Part model, mm, in its own coordinate system. A direction names the side the tool comes from. Give positions to 0.01 mm unless a question says otherwise; leave off trailing zeros. Order: outer loops, then holes, each group sorted by start corner. A loop starts at its lowest first (then second) coordinate and runs counter-clockwise, first axis right, second up. Notation, with made-up numbers: (51, 32.5) - (75, 32.5) arc R12 ccw to (75, 42.5) - close; hole circle Ø10 at (75.5, 32). An arc over 180 degrees is marked (long way). Use one line per item in the form item = value. Start each with the question number.
1. Tool access for faces 5 (the face through (29.5, 11, 39)), 6 (the face through (31.53, 26.69, 73.04)), 7 (the face through (9.84, -2.03, 57.7)): list every direction of +Z, -Z, +X, -X, +Y, -Y with a clear straight run to the whole face (end or side of a thin tool).
2. Pin check, flat tips, straight feed: P1, Ø6.5, axis at x = -9.5, z = 55.59, coming from the +Y side; P2, Ø8, axis at x = 8.5, z = 55.59, coming from the -Y side. Stop position of each tip, or through.
3. Band-saw the part on D-D, the plane x = -18.5. List the corners of the cut face in (y, z).
4. Pull direction Z, two halves, no side cores. Call faces 1 (the face through (0, -1, 80)), 2 (the face through (-33.5, 11, 39)), 3 (the face through (-31.472, 26.675, 7.004)), 4 (the face through (-31.47, 26.69, 73.04)): +Z half, -Z half, draft (parallel to the pull), parting line (faces both ways), or undercut.
5. Band-saw the part on B-B, the plane y = 9. List the corners of the cut face in (x, z), plus the area to 3 significant figures.
6. Band-saw the part on A-A, the plane x = 8.5. List the corners of the cut face in (y, z).
7. Band-saw the part on C-C, the plane z = 40. List the corners of the cut face in (x, y), plus the area to 3 significant figures.
8. Drill centre lines: line 1 (X direction, y = 14, z = 73); line 2 (Z direction, x = -31, y = 20); line 3 (Z direction, x = -18.5, y = -2.2). Where is each one in solid material? Low to high.
from build123d import *

# Parameters (mm, degrees)
SM_BASE_FLANGE_1_DEPTH   = 80
CUT_EXTRUDE_3_DEPTH      = 108.786826653
CUT_EXTRUDE_3_DEPTH_BACK = 108.786826653
SKETCH_6_R               = 48
SKETCH_6_R_2             = 2
FILLET_1_R               = 5
SKETCH_9_R               = 2.5
CUT_EXTRUDE_4_DEPTH      = 93.104560148


# Sheet-metal steps are written as plain solids
with BuildPart() as part:
    # Sketch 1 → Базовая кромка1 (new body)
    with BuildSketch(Plane.XY):
        with BuildLine():
            Line((-29.5, 27), (-29.5, 1))
            ThreePointArc((-29.5, 1), (-29.207106781, 0.292893219), (-28.5, 0))
            Line((-28.5, 0), (28.5, 0))
            ThreePointArc((28.5, 0), (29.207106781, 0.292893219), (29.5, 1))
            Line((29.5, 1), (29.5, 27))
            Line((29.5, 27), (33.5, 27))
            Line((33.5, 27), (33.5, 1))
            ThreePointArc((33.5, 1), (32.035533906, -2.535533906), (28.5, -4))
            Line((28.5, -4), (-28.5, -4))
            ThreePointArc((-28.5, -4), (-32.035533906, -2.535533906), (-33.5, 1))
            Line((-33.5, 1), (-33.5, 27))
            Line((-33.5, 27), (-29.5, 27))
        make_face()
    extrude(amount=SM_BASE_FLANGE_1_DEPTH)

    # Эскиз6 → Вырез-Вытянуть3 (cut, two sides: drawn at the far end of the back side and taken through both)
    with BuildSketch(Plane.ZY.offset(33.5).offset(-CUT_EXTRUDE_3_DEPTH_BACK)):
        with Locations((40, 62)):
            Circle(SKETCH_6_R)
        with Locations((40, 9)):
            Circle(SKETCH_6_R_2)
        with Locations((8.847381628, 19.122099298)):
            Circle(SKETCH_6_R_2)
        with Locations((71.152618372, 19.122099298)):
            Circle(SKETCH_6_R_2)
    extrude(amount=CUT_EXTRUDE_3_DEPTH + CUT_EXTRUDE_3_DEPTH_BACK, mode=Mode.SUBTRACT)

    # Скругление1
    fillet_1_edges = [part.edges().sort_by_distance(p)[0] for p in [
        (31.5, 27, 7.151864589),
        (31.5, 27, 72.848135411),
        (-31.5, 27, 7.151864589),
        (-31.5, 27, 72.848135411),
    ]]
    fillet(fillet_1_edges, radius=FILLET_1_R)

    # Эскиз9 → Вырез-Вытянуть4 (cut, through all)
    with BuildSketch(Plane.XZ.offset(4)):
        with Locations((17.5, 40)):
            Circle(SKETCH_9_R)
        with Locations((8.5, 24.411542732)):
            Circle(SKETCH_9_R)
        with Locations((-9.5, 24.411542732)):
            Circle(SKETCH_9_R)
        with Locations((-18.5, 40)):
            Circle(SKETCH_9_R)
        with Locations((-9.5, 55.588457268)):
            Circle(SKETCH_9_R)
        with Locations((8.5, 55.588457268)):
            Circle(SKETCH_9_R)
    extrude(amount=-CUT_EXTRUDE_4_DEPTH, mode=Mode.SUBTRACT)


solid = part.part
From the geometry:
q1.face_5 = +Z, -Z, +Y
q1.face_6 = +X, -X, +Y
q1.face_7 = +Y, -Y
q2.P1 = 0
q2.P2 = -4
q3.outline = (-4, 0) - (0, 0) - (0, 37.5) - (-4, 37.5) - close; (-4, 42.5) - (0, 42.5) - (0, 80) - (-4, 80) - close
q4.face_1 = +Z half
q4.face_2 = draft
q4.face_3 = undercut
q4.face_4 = undercut
q5.outline = (-33.5, 0) - (-29.5, 0) - (-29.5, 38) - (-33.5, 38) - close; (-33.5, 42) - (-29.5, 42) - (-29.5, 80) - (-33.5, 80) - close; (29.5, 0) - (33.5, 0) - (33.5, 38) - (29.5, 38) - close; (29.5, 42) - (33.5, 42) - (33.5, 80) - (29.5, 80) - close
q5.area = 608 mm²
q6.outline = (-4, 0) - (0, 0) - (0, 21.91) - (-4, 21.91) - close; (-4, 26.91) - (0, 26.91) - (0, 53.09) - (-4, 53.09) - close; (-4, 58.09) - (0, 58.09) - (0, 80) - (-4, 80) - close
q7.outline = (-33.5, 1) arc R5 ccw to (-28.5, -4) - (-21, -4) - (-21, 0) - (-28.5, 0) arc R1 cw to (-29.5, 1) - (-29.5, 7) - (-33.5, 7) - close; (-33.5, 11) - (-29.5, 11) - (-29.5, 14) - (-33.5, 14) - close; (-16, -4) - (15, -4) - (15, 0) - (-16, 0) - close; (20, -4) - (28.5, -4) arc R5 ccw to (33.5, 1) - (33.5, 7) - (29.5, 7) - (29.5, 1) arc R1 cw to (28.5, 0) - (20, 0) - close; (29.5, 11) - (33.5, 11) - (33.5, 14) - (29.5, 14) - close
q7.area = 298 mm²
q8.line_1 = -33.5 to -29.5, 29.5 to 33.5
q8.line_2 = 0 to 7.05, 10.64 to 16.76, 63.24 to 69.36, 72.95 to 80
q8.line_3 = 0 to 37.5, 42.5 to 80
